Here's how the part is built. I have some questions about the finished solid (model axes, mm). A direction names the side the tool comes from. Coordinates: 2 decimals unless noted, no trailing zeros. Loops run counter-clockwise (first coordinate to the right, second up) from the corner with the lowest first, then second, coordinate; pieces in that order, holes last.
from build123d import *

# Parameters (mm, degrees)
F0_W     = 12
F0_H     = 14.75
F1_DEPTH = 34
F2_W     = 8
F2_H     = 10.75
F3_DEPTH = 36
F5_D     = 5


with BuildPart() as f1:
    # F0 (on Top) → F1 (new body)
    with BuildSketch(Plane.XY):
        Rectangle(F0_W, F0_H)
    extrude(amount=-F1_DEPTH)

    # F2 (on face) → F3 (cut)
    with BuildSketch(Plane.XY):
        Rectangle(F2_W, F2_H)
    extrude(amount=-F3_DEPTH, mode=Mode.SUBTRACT)

    # F5 (through all)
    with Locations(Plane.XZ.offset(7.375)):
        with Locations((0, -8)):
            Hole(F5_D / 2)


solid = f1.part
Q1. Suppose I cut it at A-A on x = -1.5. Write out the boundary of the cut face in (y, z) (3 decimals), and give its area (3 significant figures).
Q2. Suppose I cut it at C-C on z = -23.5. Write out the boundary of the cut face in (x, y) (3 decimals), and give its area (3 significant figures).
Q3. Suppose I cut it at B-B on y = -0.25. Write out the boundary of the cut face in (x, z).
Q4. We'd pull the mould along Z, two halves only. Please class faces 3 (the flat face through (6, 0, -17)), 4 (the cylindrical face through (0.54, 6.39, -10.44)), 5 (the flat face through (-5, 0, -34)): pulls with the +Z half, pulls with the -Z half, needs draft (parallel to the pull), parting line crosses it, or undercut.
Q5. Please list where these lines run through material, in increasing order: probe 1 along Y at (x, z) = (3.75, -11.5) (3 decimals); probe 2 along Z at (x, y) = (0, 6.3); probe 3 along X at (y, z) = (2, -11).
Q6. Suppose I cut it at D-D on x = 3.5. Write out the boundary of the cut face in (y, z) (3 decimals), and give its area (3 significant figures).
Q7. For faces 1 (the flat face through (-4, 0, -17)), 2 (the cylindrical face through (0.54, -6.36, -10.44)), which set-ups out of +Z, -Z, +X, -X, +Y, -Y let a thin tool reach every point of the face, with its end or its side?
Check values:
1. outline: (-7.375, -34) - (-5.375, -34) - (-5.375, -10) - (-7.375, -10) - close; (-7.375, -6) - (-5.375, -6) - (-5.375, 0) - (-7.375, 0) - close; (5.375, -34) - (7.375, -34) - (7.375, -10) - (5.375, -10) - close; (5.375, -6) - (7.375, -6) - (7.375, 0) - (5.375, 0) - close
1. area: 120 mm2
2. outline: (-6, -7.375) - (6, -7.375) - (6, 7.375) - (-6, 7.375) - close; hole (-4, -5.375) - (4, -5.375) - (4, 5.375) - (-4, 5.375) - close
2. area: 91.0 mm2
3. outline: (-6, -34) - (-4, -34) - (-4, 0) - (-6, 0) - close; (4, -34) - (6, -34) - (6, 0) - (4, 0) - close
4. face 3: needs draft
4. face 4: undercut
4. face 5: pulls with the -Z half
5. probe 1: y = -7.375 to -5.375, 5.375 to 7.375
5. probe 2: z = -34 to -10.5, -5.5 to 0
5. probe 3: x = -6 to -4, 4 to 6
6. outline: (-7.375, -34) - (-5.375, -34) - (-5.375, 0) - (-7.375, 0) - close; (5.375, -34) - (7.375, -34) - (7.375, 0) - (5.375, 0) - close
6. area: 136 mm2
7. face 1: +Z, -Z
7. face 2: +Y, -Y
